from build123d import *

# Parameters (mm, degrees)
ESQUISSE1_R             = 10
ESQUISSE1_R_2           = 5
BOSS_EXTRU_1_DEPTH      = 5
ESQUISSE2_W             = 5
ESQUISSE2_H             = 7
BOSS_EXTRU_2_DEPTH      = 5
ESQUISSE3_R             = 1
ENL_V_MAT_EXTRU_1_DEPTH = 10


with BuildPart() as part:
    # Esquisse1 → Boss.-Extru.1 (new body)
    with BuildSketch(Plane.XY):
        Circle(ESQUISSE1_R)
        Circle(ESQUISSE1_R_2, mode=Mode.SUBTRACT)
    extrude(amount=BOSS_EXTRU_1_DEPTH)

    # Esquisse2 → Boss.-Extru.2 (add)
    with BuildSketch(Plane.XY.offset(5)):
        with Locations((0, 11.5)):
            Rectangle(ESQUISSE2_W, ESQUISSE2_H)
    extrude(amount=-BOSS_EXTRU_2_DEPTH)

    # Esquisse3 → Enlèv. mat.-Extru.1 (cut)
    with BuildSketch(Plane(origin=(-2.5, 0, 0), x_dir=(0, -1, 0), z_dir=(-1, 0, 0))):
        with Locations((-12.345891544, 2.487364075)):
            Circle(ESQUISSE3_R)
    extrude(amount=-ENL_V_MAT_EXTRU_1_DEPTH, mode=Mode.SUBTRACT)


solid = part.part
Verification items for the finished model (mm, model axes). A direction names the side the tool comes from. Coordinates: 2 decimals unless noted, no trailing zeros. Order: outer loops, then holes, each group sorted by start corner. A loop starts at its lowest first (then second) coordinate and runs counter-clockwise, first axis right, second up. Notation, with made-up numbers: M 56,84.5 L 85,84.5 A22 ccw 85,108.5 Z; hole C -3.75,83 d3. An arc over 180 degrees is marked long. One line per item, written item: value. Start each with the question number.
Item 1: Depth check by flat-ended pin: P1, Ø5, axis at x = 7, y = -7.5, coming from the +Z side; P2, Ø1.5, axis at y = 12.5, z = 3.5, coming from the +X side; P3, Ø2.5, axis at y = 12.35, z = 2.49, coming from the -X side; P4, Ø6, axis at x = 0, y = 0, coming from the +Z side. Enter the tip coordinate at first touch or a pass-through.
Item 2: Access from +Z, -Z, +X, -X, +Y, -Y to the whole of each face (thin tool, end or side, straight path). Record for faces 1 (the flat face through (-2.5, 12, 4)), 2 (the flat face through (2.5, 12, 4)), 3 (the flat face through (-0.1, 5.5, 5)).
Item 3: Sectioned sample at C-C on z = 3.1. Record the cut outline in (x, y), then the cut area to 3 significant figures.
Item 4: Sectioned sample at A-A on y = 0. Record the cut outline in (x, z).
Item 5: Mould release check, pull along Y, two halves, no side actions. Record for faces 4 (the flat face through (-0.1, 5.5, 0)), 5 (the cylindrical face through (-0.035, 11.392, 2.788)), 6 (the cylindrical face through (0, -10, 2)), 7 (the flat face through (0, 15, 3)): pulls with the +Y half, pulls with the -Y half, needs draft (parallel to the pull), parting line crosses it, or undercut.
Item 6: Thickness scan on probe 1 along X at (y, z) = (3.5, 4.4); probe 2 along X at (y, z) = (2, 3.3); probe 3 along X at (y, z) = (10.5, 3.1). Record the ranges inside material, lowest first.
Item 7: Sectioned sample at D-D on x = -4.5. Record the cut outline in (y, z), then the cut area to 3 significant figures.
Item 8: Sectioned sample at B-B on x = 0. Record the cut outline in (y, z).
Calculated:
1. P1: z = 5
1. P2: x = 2.5
1. P3: x = -2.5
1. P4: through
2. face 1: +Z, -Z, -X, +Y
2. face 2: +Z, -Z, +X, +Y
2. face 3: +Z, +X, -X, +Y, -Y
3. outline: M -2.5,9.68 A10 ccw long 2.5,9.68 L 2.5,11.56 L -2.5,11.56 Z; M -2.5,13.14 L 2.5,13.14 L 2.5,15 L -2.5,15 Z; hole C 0,0 d10
3. area: 253 mm^2
4. outline: M -10,0 L -5,0 L -5,5 L -10,5 Z; M 5,0 L 10,0 L 10,5 L 5,5 Z
5. face 4: needs draft
5. face 5: undercut
5. face 6: parting line crosses it
5. face 7: pulls with the +Y half
6. probe 1: -9.37 to -3.57, 3.57 to 9.37
6. probe 2: -9.8 to -4.58, 4.58 to 9.8
6. probe 3: -2.5 to 2.5
7. outline: M -8.93,0 L -2.18,0 L -2.18,5 L -8.93,5 Z; M 2.18,0 L 8.93,0 L 8.93,5 L 2.18,5 Z
7. area: 67.5 mm^2
8. outline: M -10,0 L -5,0 L -5,5 L -10,5 Z; M 5,0 L 15,0 L 15,5 L 5,5 Z; hole C 12.35,2.49 d2
